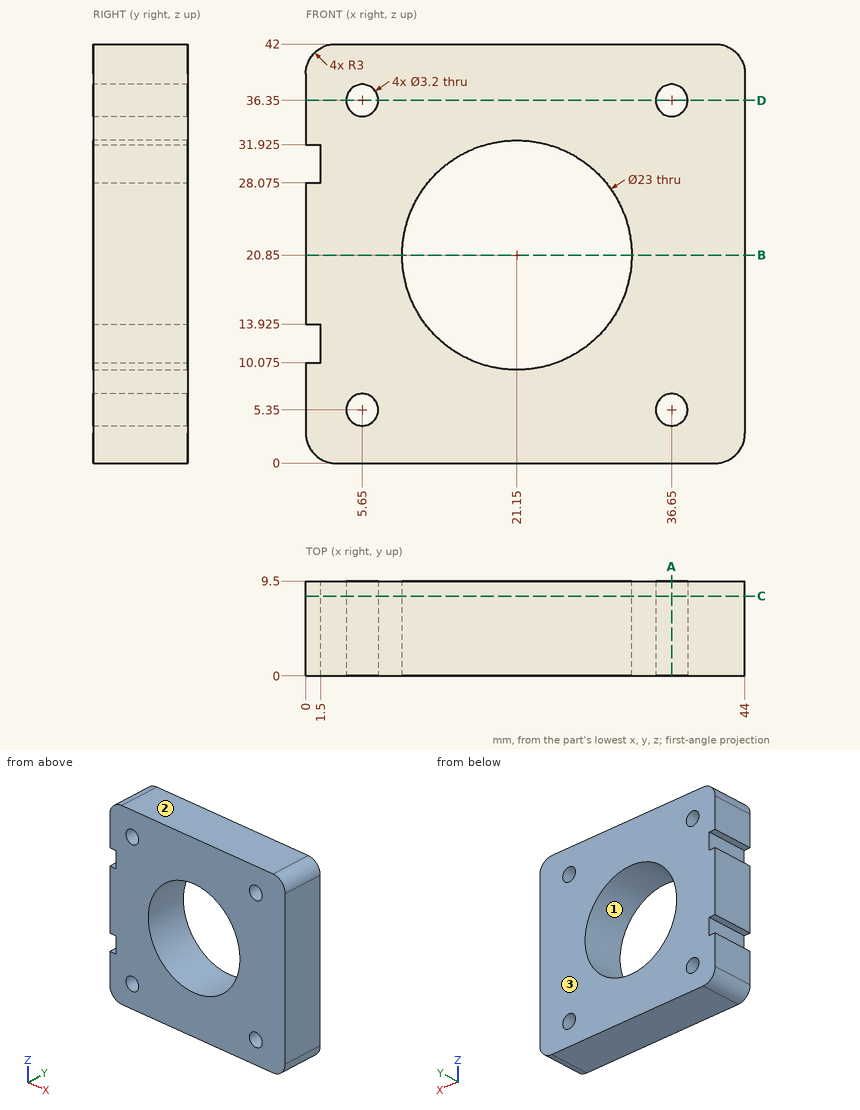
Drawing for the job (mm, zero at the part's lowest x, y, z). Give positions to 0.01 mm unless a question says otherwise; leave off trailing zeros. Loops run counter-clockwise (first coordinate to the right, second up) from the corner with the lowest first, then second, coordinate; pieces in that order, holes last. Notation, with made-up numbers: M 27,48.25 L 32,48.25 A8 cw 32,61.25 Z; hole C -17.75,-10 d11. An arc over 180 degrees is marked long. One line per question, with ' | ' between items. Start each with the question number.
1. Probe L1, parallel to X at y = 7.5, z = 5.35; L2, parallel to X at y = 8.75, z = 4; L3, parallel to X at y = 3.5, z = 20.85. List the from-to ranges inside material, lowest first. Write a range as from..to.
2. Flat gauge pins, fed straight in: pin 1 (0.8 mm diameter, centred on x = 1, y = 3.5, fed in from +Z); pin 2 (1.5 mm diameter, centred on x = 33.5, z = 13, fed in from -Y); pin 3 (1.2 mm diameter, centred on y = 3.5, z = 12, fed in from -X). Where does each tip first touch, or does it go through?
3. Two-plate mould, pull along Z, no slides. Class the marked faces 1, 2 and 3: pulls with the +Z half, pulls with the -Z half, needs draft (parallel to the pull), parting line crosses it, or undercut.
4. Saw through at D-D on z = 36.35. Give the cut face in (x, y), plus the area to 3 significant figures.
5. Saw through at A-A on x = 36.65. Give the cut face in (y, z).
6. Saw through at B-B on z = 20.85. Give the cut face in (x, y).
7. Saw through at C-C on y = 8. Give the cut face in (x, z) (3 decimals), plus the area to 3 significant figures.
Result sheet:
1) L1: x = 0..4.05, 7.25..35.05, 38.25..44 | L2: x = 0..4.79, 6.51..35.79, 37.51..44 | L3: x = 0..9.65, 32.65..44
2) pin 1: stops at z = 41.54 | pin 2: stops at y = 0 | pin 3: stops at x = 1.5
3) face 1: undercut | face 2: pulls with the +Z half | face 3: needs draft
4) outline: M 0,0 L 4.05,0 L 4.05,9.5 L 0,9.5 Z; M 7.25,0 L 35.05,0 L 35.05,9.5 L 7.25,9.5 Z; M 38.25,0 L 44,0 L 44,9.5 L 38.25,9.5 Z | area: 357 mm^2
5) outline: M 0,0 L 9.5,0 L 9.5,3.75 L 0,3.75 Z; M 0,6.95 L 9.5,6.95 L 9.5,34.75 L 0,34.75 Z; M 0,37.95 L 9.5,37.95 L 9.5,42 L 0,42 Z
6) outline: M 0,0 L 9.65,0 L 9.65,9.5 L 0,9.5 Z; M 32.65,0 L 44,0 L 44,9.5 L 32.65,9.5 Z
7) outline: M 0,3 A3 ccw 3,0 L 41,0 A3 ccw 44,3 L 44,39 A3 ccw 41,42 L 3,42 A3 ccw 0,39 L 0,31.925 L 1.5,31.925 L 1.5,28.075 L 0,28.075 L 0,13.925 L 1.5,13.925 L 1.5,10.075 L 0,10.075 Z; hole C 5.65,5.35 d3.2; hole C 5.65,36.35 d3.2; hole C 21.15,20.85 d23; hole C 36.65,5.35 d3.2; hole C 36.65,36.35 d3.2 | area: 1,380 mm^2
